```python
from build123d import *

# Parameters (mm, degrees)
SKETCH_1_W          = 64
SKETCH_1_H          = 15
EXTRUDE_1_DEPTH     = 7
SKETCH_2_W          = 40
SKETCH_2_H          = 15
EXTRUDE_2_DEPTH     = 23
SKETCH_3_R          = 5
CUT_EXTRUDE_1_DEPTH = 20
SKETCH_4_W          = 40
SKETCH_4_H          = 3
CUT_EXTRUDE_2_DEPTH = 10
HOLE_WIZARD_M5_1_D  = 5
SKETCH_8_R          = 3.5
CUT_EXTRUDE_3_DEPTH = 4
HOLE_WIZARD_M5_2_D  = 5
CUT_EXTRUDE_5_DEPTH = 2
FILLET_1_R          = 0.8


with BuildPart() as part:
    # 草图1 → 凸台-拉伸1 (new body)
    with BuildSketch(Plane(origin=(0, 0, 0), x_dir=(1, 0, 0), z_dir=(0, 1, 0))):
        Rectangle(SKETCH_1_W, SKETCH_1_H)
    extrude(amount=EXTRUDE_1_DEPTH)

    # 草图2 → 凸台-拉伸2 (add)
    with BuildSketch(Plane(origin=(0, 7, 0), x_dir=(1, 0, 0), z_dir=(0, 1, 0))):
        Rectangle(SKETCH_2_W, SKETCH_2_H)
    extrude(amount=EXTRUDE_2_DEPTH)

    # 草图3 → 切除-拉伸1 (cut)
    with BuildSketch(Plane(origin=(0, 30, 0), x_dir=(1, 0, 0), z_dir=(0, 1, 0))):
        with Locations(Location((0, 0, 0), (0, 0, 270))):
            Circle(SKETCH_3_R)
    extrude(amount=-CUT_EXTRUDE_1_DEPTH, mode=Mode.SUBTRACT)

    # 草图4 → 切除-拉伸2 (cut)
    with BuildSketch(Plane(origin=(0, 30, 0), x_dir=(1, 0, 0), z_dir=(0, 1, 0))):
        Rectangle(SKETCH_4_W, SKETCH_4_H)
    extrude(amount=-CUT_EXTRUDE_2_DEPTH, mode=Mode.SUBTRACT)

    # M5 螺纹孔的螺纹孔钻头1 (through all)
    with Locations(Plane.XY.offset(7.5)):
        with Locations((-14, 24.5), (14, 24.5)):
            Hole(HOLE_WIZARD_M5_1_D / 2)

    # 草图8 → 切除-拉伸3 (cut)
    with BuildSketch(Plane(origin=(0, 7, 0), x_dir=(1, 0, 0), z_dir=(0, 1, 0))):
        with Locations(Location((-26, 0, 0), (0, 0, 270))):
            Circle(SKETCH_8_R)
    cut_extrude_3 = extrude(amount=-CUT_EXTRUDE_3_DEPTH, mode=Mode.SUBTRACT)

    # M5 螺纹孔的螺纹孔钻头2 (through all)
    with Locations(Plane(origin=(0, 3, 0), x_dir=(1, 0, 0), z_dir=(0, 1, 0))):
        with Locations((-26, 0)):
            hole_wizard_m5_2 = Hole(HOLE_WIZARD_M5_2_D / 2)

    # 镜向1: 切除-拉伸3, M5 螺纹孔的螺纹孔钻头2 across plane
    add(cut_extrude_3.mirror(Plane(origin=(0, 0, 0), x_dir=(0, 0, 1), z_dir=(1, 0, 0))), mode=Mode.SUBTRACT)
    add(hole_wizard_m5_2.mirror(Plane(origin=(0, 0, 0), x_dir=(0, 0, 1), z_dir=(1, 0, 0))), mode=Mode.SUBTRACT)

    # 草图12 → 切除-拉伸5 (cut)
    with BuildSketch(Plane.XY.offset(7.5)):
        Polygon((-14, 19.881197846), (-10, 22.190598923), (-10, 26.809401077), (-14, 29.118802154), (-18, 26.809401077), (-18, 22.190598923), align=None)
        Polygon((14, 19.881197846), (18, 22.190598923), (18, 26.809401077), (14, 29.118802154), (10, 26.809401077), (10, 22.190598923), align=None)
    extrude(amount=-CUT_EXTRUDE_5_DEPTH, mode=Mode.SUBTRACT)

    # 圆角1
    fillet_1_edges = [part.edges().sort_by_distance(p)[0] for p in [
        (-32, 7, 0),
        (-26, 7, -7.5),
        (26, 7, 7.5),
        (20, 7, 0),
        (20, 18.5, 7.5),
        (20, 18.5, -7.5),
        (-20, 7, 0),
        (-20, 18.5, -7.5),
        (-26, 7, 7.5),
        (-20, 18.5, 7.5),
        (20, 30, 4.5),
        (0, 30, -7.5),
        (-20, 30, -4.5),
        (0, 30, 7.5),
        (20, 30, -4.5),
        (-20, 30, 4.5),
        (32, 7, 0),
        (0, 0, 7.5),
        (-32, 0, 0),
        (0, 0, -7.5),
        (32, 0, 0),
        (26, 7, -7.5),
    ]]
    fillet(fillet_1_edges, radius=FILLET_1_R)


solid = part.part
```
Could you check a few things on this model? Use its own coordinates, in mm. A direction names the side the tool comes from. Round coordinates to 2 decimals unless told otherwise and drop trailing zeros. Loops run counter-clockwise (first coordinate to the right, second up) from the corner with the lowest first, then second, coordinate; pieces in that order, holes last. Notation, with made-up numbers: (-7.5, 7.5) - (19.5, 7.5) arc R24 ccw to (19.5, 30.5) - close; hole circle Ø3 at (63, -18). An arc over 180 degrees is marked (long way). Use CSV: the item, a comma, the result in double quotes.
Item 1: If we section it at C-C on x = 26: List the corners of the cut face in (y, z) for me, then the cut area to 3 significant figures.
Here are the results:
outline,"(0, -6.7) arc R0.8 ccw to (0.8, -7.5) - (6.2, -7.5) arc R0.8 ccw to (7, -6.7) - (7, -3.5) - (3, -3.5) - (3, -2.5) - (0, -2.5) - close; (0, 2.5) - (3, 2.5) - (3, 3.5) - (7, 3.5) - (7, 6.7) arc R0.8 ccw to (6.2, 7.5) - (0.8, 7.5) arc R0.8 ccw to (0, 6.7) - close"
area,"61.5 mm²"
Item 2: If we section it at A-A on z = -6: List the corners of the cut face in (x, y) for me.
Here are the results:
outline,"(-32, 0.8) arc R0.8 ccw to (-31.2, 0) - (31.2, 0) arc R0.8 ccw to (32, 0.8) - (32, 6.2) arc R0.8 ccw to (31.2, 7) - (20.8, 7) arc R0.8 cw to (20, 7.8) - (20, 29.2) arc R0.8 ccw to (19.2, 30) - (-19.2, 30) arc R0.8 ccw to (-20, 29.2) - (-20, 7.8) arc R0.8 cw to (-20.8, 7) - (-31.2, 7) arc R0.8 ccw to (-32, 6.2) - close; hole circle Ø5 at (-14, 24.5); hole circle Ø5 at (14, 24.5)"
Item 3: If we mould it in two halves opening along Y, with no side actions, what happens to faces 6 (the flat face through (-0.3, 30, -5.3)), 7 (the flat face through (12.2, 22.5, 5.5)), 8 (the cylindrical face through (-14, 27, -5)), 9 (the cylindrical face through (23.5, 1.5, -0.1))? For each: pulls with the +Y half, pulls with the -Y half, needs draft (parallel to the pull), parting line crosses it, or undercut.
Here are the results:
face 6,"pulls with the +Y half"
face 7,"undercut"
face 8,"undercut"
face 9,"needs draft"
Item 4: For faces 1 (the flat face through (15.97, 21.02, 6.51)), 2 (the flat face through (32, 3, 0)), 3 (the flat face through (11, 25, -1.5)), 4 (the flat face through (-0.3, 30, 5.2)), 5 (the cylindrical face through (-1.915, 20.14, 4.619)), which set-ups out of +Z, -Z, +X, -X, +Y, -Y let a thin tool reach every point of the face, with its end or its side?
Here are the results:
face 1,"+Z"
face 2,"+Z, -Z, +X, +Y, -Y"
face 3,"+X, -X, +Y"
face 4,"+Z, -Z, +X, -X, +Y"
face 5,"+Y"
Item 5: If we section it at B-B on y = 13: List the corners of the cut face in (x, z) for me, then the cut area to 3 significant figures.
Here are the results:
outline,"(-20, -6.7) arc R0.8 ccw to (-19.2, -7.5) - (19.2, -7.5) arc R0.8 ccw to (20, -6.7) - (20, 6.7) arc R0.8 ccw to (19.2, 7.5) - (-19.2, 7.5) arc R0.8 ccw to (-20, 6.7) - close; hole circle Ø10 at (0, 0)"
area,"521 mm²"
Item 6: I need wall thicknesses on L1, parallel to X at y = 16, z = -1.5; L2, parallel to X at y = 4.45, z = 0; L3, parallel to Z at x = -16.5, y = 24. Which ranges of each line are inside material? Lowest first, please. Write a range as [from, to].
Here are the results:
L1,"x = [-20, -4.77], [4.77, 20]"
L2,"x = [-32, -29.5], [-22.5, 22.5], [29.5, 32]"
L3,"z = [-7.5, -1.5], [1.5, 5.5]"
Item 7: Will these pins go through, and if not, where does the flat tip stop? pin 1 (2 mm diameter, centred on y = 25, z = 7, fed in from +X); pin 2 (1.6 mm diameter, centred on y = 25, z = 6.5, fed in from -X); pin 3 (5 mm diameter, centred on x = -27, z = -1.5, fed in from +Y).
Here are the results:
pin 1,"stops at x = 20"
pin 2,"stops at x = -20"
pin 3,"stops at y = 7"
Item 8: If we section it at D-D on z = 0: Count the separate pieces of the cut face and the enclosed holes in it, then the cut area to 3 significant figures.
Here are the results:
separate pieces,"3"
enclosed holes,"0"
area,"782 mm²"
